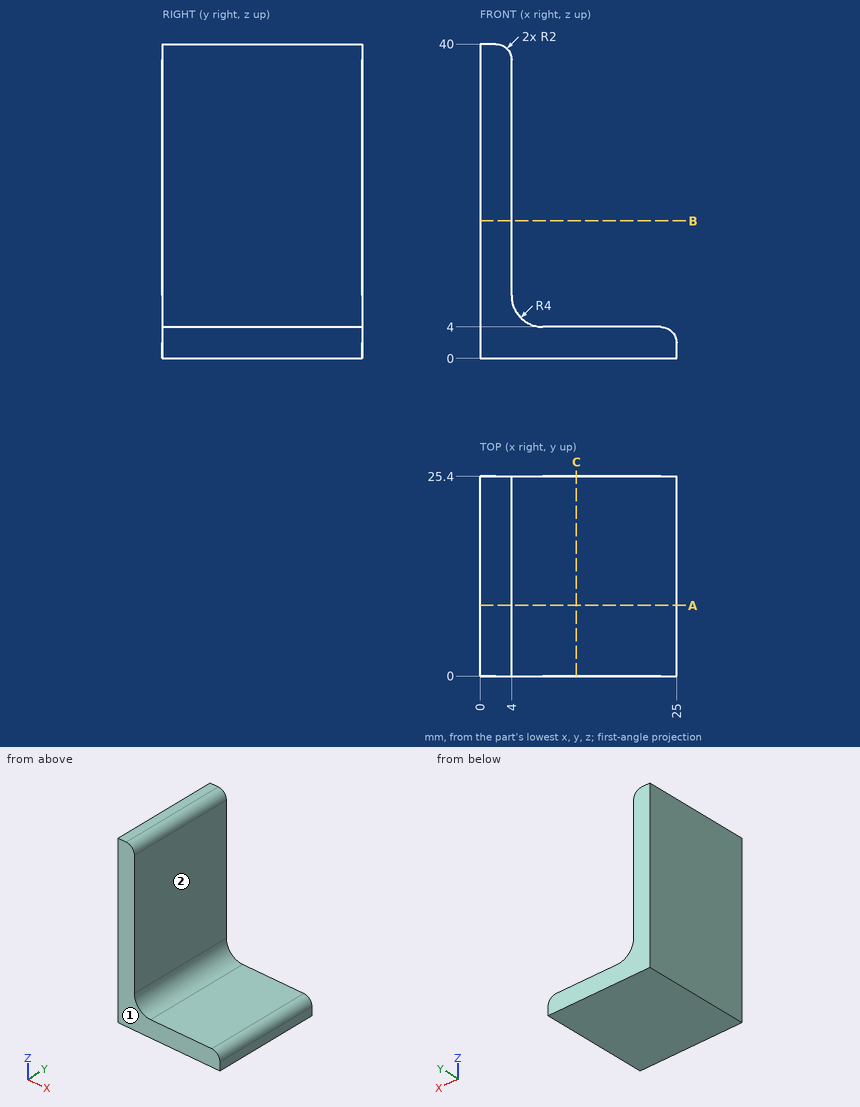
Input: dimensioned drawing with shaded views. Units: mm. Origin: part minimum x, y, z. A direction names the side the tool comes from. Round coordinates to 2 decimals unless told otherwise and drop trailing zeros. Order: outer loops, then holes, each group sorted by start corner. A loop starts at its lowest first (then second) coordinate and runs counter-clockwise, first axis right, second up.
1. Cut plane A-A, the plane y = 9. Output: boundary loops of the cut face in (x, z).
The answers:
outline: (0, 0) - (25, 0) - (25, 2) arc R2 ccw to (23, 4) - (8, 4) arc R4 cw to (4, 8) - (4, 38) arc R2 ccw to (2, 40) - (0, 40) - close
2. Cut plane C-C, the plane x = 12.25. Output: boundary loops of the cut face in (y, z), then the cut area to 3 significant figures.
The answers:
outline: (0, 0) - (25.4, 0) - (25.4, 4) - (0, 4) - close
area: 102 mm2
3. Cut plane B-B, the plane z = 17.5. Output: boundary loops of the cut face in (x, y), then the cut area to 3 significant figures.
The answers:
outline: (0, 0) - (4, 0) - (4, 25.4) - (0, 25.4) - close
area: 102 mm2
4. Pin query (flat end, axial travel): P1, Ø7.5, axis at y = 16.5, z = 26.5, coming from the +X side; P2, Ø8, axis at x = 13, y = 6, coming from the +Z side; P3, Ø2, axis at y = 21.5, z = 4, coming from the +X side. Return the tip coordinate at first contact, or that it passes through.
The answers:
P1: stops at x = 4
P2: stops at z = 4
P3: stops at x = 24.73
5. Set-up query: the marked faces 1 and 2. Return all of +Z, -Z, +X, -X, +Y, -Y with unobstructed straight access to the full face (end or side cutting, diameter ignored); none if empty.
The answers:
face 1: +Z, -Z, +X, -X, -Y
face 2: +Z, +X, +Y, -Y
6. Material intervals for line 1 (Z direction, x = 10, y = 12); line 2 (Z direction, x = 4.5, y = 10.25), sorted ascending.
The answers:
line 1: z = 0 to 4
line 2: z = 0 to 6.06
